```python
from build123d import *

# Parameters (mm, degrees)
F0_W     = 20
F0_H     = 20
F1_DEPTH = 25
F2_W     = 16.8
F2_H     = 16.8
F3_DEPTH = 20
F4_SIZE  = 1
F5_R     = 9.99999
F7_D     = 8.2
F7_DEPTH = 35
F7_TIP   = 2.463528538


# Not quite as in the source:
# - a fillet or chamfer is up to 0.001 mm smaller than in the source, because OpenCascade refuses the exact size


with BuildPart() as f1:
    # F0 (on Top) → F1 (new body)
    with BuildSketch(Plane.XY):
        with Locations((15, 10)):
            Rectangle(F0_W, F0_H)
    extrude(amount=F1_DEPTH)

    # F2 (on face) → F3 (join)
    with BuildSketch(Plane.XY.offset(25)):
        with Locations((15, 10)):
            Rectangle(F2_W, F2_H)
    extrude(amount=F3_DEPTH)

    # F4
    f4_edges = [f1.edges().sort_by_distance(p)[0] for p in [
        (6.6, 18.4, 35),
        (6.6, 10, 45),
        (15, 18.4, 45),
        (23.4, 18.4, 35),
        (23.4, 10, 45),
        (15, 1.6, 45),
        (6.6, 1.6, 35),
        (23.4, 1.6, 35),
    ]]
    chamfer(f4_edges, length=F4_SIZE)

    # F5 (radius 10 in the source; OpenCascade refuses exactly that, so slightly less here)
    f5_edges = [f1.edges().sort_by_distance(p)[0] for p in [
        (15, 0, 0),
        (15, 20, 0),
    ]]
    fillet(f5_edges, radius=F5_R)

    # F7
    with Locations(Plane.YZ.offset(25)):
        with Locations((10, 10)):
            Hole(F7_D / 2, depth=F7_DEPTH)
            with Locations((0, 0, -(F7_DEPTH + F7_TIP / 2))):  # 118° drill point
                Cone(0, F7_D / 2, F7_TIP, mode=Mode.SUBTRACT)


solid = f1.part
```
Input: part model. Units: mm. Frame: model coordinates. A direction names the side the tool comes from. Coordinates: 2 decimals unless noted, no trailing zeros. Loops run counter-clockwise (first coordinate to the right, second up) from the corner with the lowest first, then second, coordinate; pieces in that order, holes last.
Q1. Section B-B, the plane y = 9.5. Return the cut outline in (x, z), and give its area (3 significant figures).
Results are:
outline: (5, 0.01) - (25, 0.01) - (25, 5.93) - (5, 5.93) - close; (5, 14.07) - (25, 14.07) - (25, 25) - (23.4, 25) - (23.4, 44) - (22.4, 45) - (7.6, 45) - (6.6, 44) - (6.6, 25) - (5, 25) - close
area: 672 mm2
Q2. Mould query, pull axis Z, two halves, no side actions, for faces 6 (the cylindrical face through (15.14, 2.85, 3.01)), 7 (the flat face through (15, 10, 45)), 8 (the cylindrical face through (14.86, 14.096, 10.18)). Classes: +Z half, -Z half, draft (parallel to the pull), parting line (faces both ways), or undercut.
Results are:
face 6: -Z half
face 7: +Z half
face 8: undercut
Q3. Set-up query: faces 1 (the flat face through (7.1, 2.1, 34.4)), 2 (the flat face through (6.6, 10, 34)), 3 (the flat face through (15, 1.6, 34)), 4 (the flat face through (22.9, 2.1, 34.4)), 5 (the flat face through (15, 18.4, 34)). Return all of +Z, -Z, +X, -X, +Y, -Y with unobstructed straight access to the full face (end or side cutting, diameter ignored); none if empty.
Results are:
face 1: +Z, -X, -Y
face 2: +Z, -X, +Y, -Y
face 3: +Z, +X, -X, -Y
face 4: +Z, +X, -Y
face 5: +Z, +X, -X, +Y
Q4. Contact query for flat-ended pins moving along their axis: pin 1 (4.5 mm diameter, centred on x = 11.5, z = 31, fed in from -Y); pin 2 (4.5 mm diameter, centred on x = 16.5, z = 35.5, fed in from +Y). Output: stop coordinate, or through.
Results are:
pin 1: stops at y = 1.6
pin 2: stops at y = 18.4
Q5. Line query: line 1 along Z through (x, y) = (10, 10); line 2 along Y through (x, z) = (16, 29.5); line 3 along Z through (x, y) = (18.5, 6.5). Output: solid intervals per line, ascending.
Results are:
line 1: z = 0 to 5.9, 14.1 to 45
line 2: y = 1.6 to 18.4
line 3: z = 0.63 to 7.86, 12.14 to 45
Q6. Section C-C, the plane z = 31. Return the cut outline in (x, y).
Results are:
outline: (6.6, 2.6) - (7.6, 1.6) - (22.4, 1.6) - (23.4, 2.6) - (23.4, 17.4) - (22.4, 18.4) - (7.6, 18.4) - (6.6, 17.4) - close
